Check sheet for the drawn part. Datum: minimum x, y, z corner. Units: mm. A direction names the side the tool comes from. Coordinates: 2 decimals unless noted, no trailing zeros. Loops run counter-clockwise (first coordinate to the right, second up) from the corner with the lowest first, then second, coordinate; pieces in that order, holes last.
Q1. Material ranges on probe 1 along Y at (x, z) = (10, 1.4); probe 2 along Z at (x, y) = (5, 16.5); probe 3 along Y at (x, z) = (3, 0.55), recorded low to high.
Q2. Sectioned sample at D-D (z = 1.75). Enter the section's corners in (x, y), then the cut area to 3 significant figures.
Q3. Mould release check, pull along X, two halves, no side actions. Record for the marked faces 1, 2 and 3: +X half, -X half, draft (parallel to the pull), parting line (faces both ways), or undercut.
Q4. Sectioned sample at C-C (y = 16.5). Enter the section's corners in (x, z).
Q5. Sectioned sample at A-A (x = 10). Enter the section's corners in (y, z), then the cut area to 3 significant figures.
Q6. Go/stop test with flat-tipped pins: P1, Ø2.5, axis at x = 10, y = 10, coming from the +Z side; P2, Ø1, axis at y = 14.5, z = 2, coming from the -X side. Record where each tip stops, or that it passes through.
Q7. Access from +Z, -Z, +X, -X, +Y, -Y to the whole of each face (thin tool, end or side, straight path). Record for the marked faces 4 and 5.
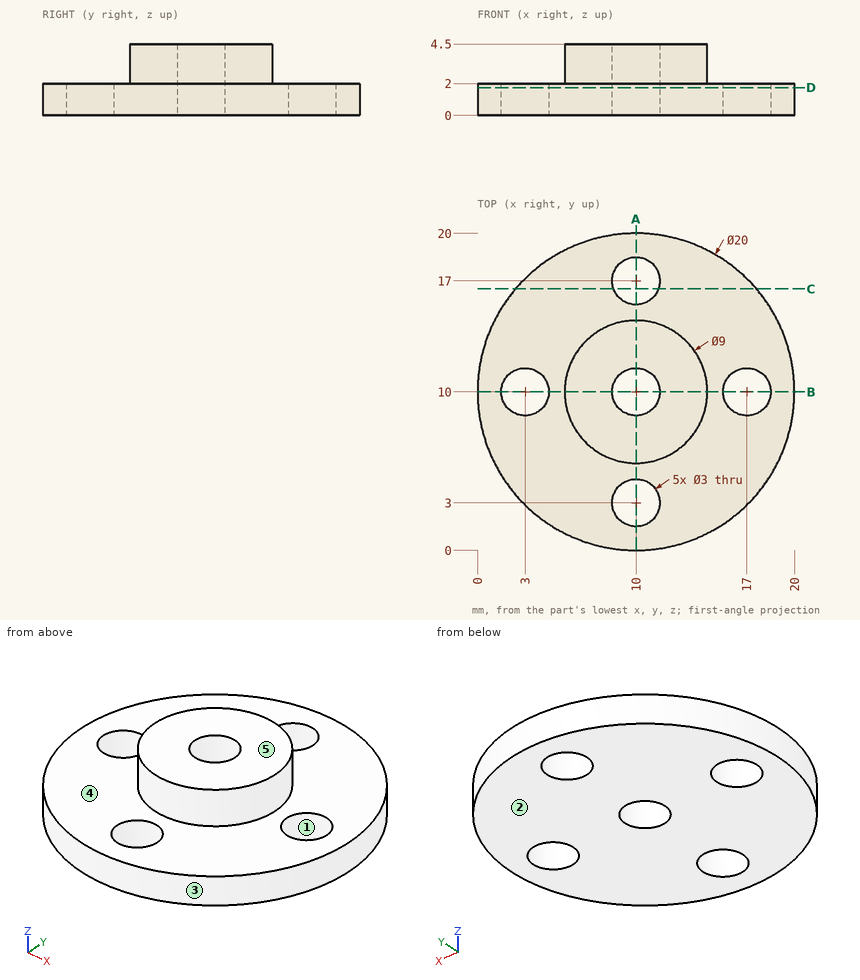
Geometry check:
1. probe 1: y = 0 to 1.5, 4.5 to 8.5, 11.5 to 15.5, 18.5 to 20
1. probe 2: z = 0 to 2
1. probe 3: y = 2.86 to 8.5, 11.5 to 17.14
2. outline: circle Ø20 at (10, 10); hole circle Ø3 at (3, 10); hole circle Ø3 at (10, 3); hole circle Ø3 at (10, 10); hole circle Ø3 at (10, 17); hole circle Ø3 at (17, 10)
2. area: 279 mm2
3. face 1: undercut
3. face 2: draft
3. face 3: parting line
4. outline: (2.4, 0) - (8.59, 0) - (8.59, 2) - (2.4, 2) - close; (11.41, 0) - (17.6, 0) - (17.6, 2) - (11.41, 2) - close
5. outline: (0, 0) - (1.5, 0) - (1.5, 2) - (0, 2) - close; (4.5, 0) - (8.5, 0) - (8.5, 4.5) - (5.5, 4.5) - (5.5, 2) - (4.5, 2) - close; (11.5, 0) - (15.5, 0) - (15.5, 2) - (14.5, 2) - (14.5, 4.5) - (11.5, 4.5) - close; (18.5, 0) - (20, 0) - (20, 2) - (18.5, 2) - close
5. area: 37.0 mm2
6. P1: passes through
6. P2: stops at x = 0.83
7. face 4: +Z
7. face 5: +Z, +X, -X, +Y, -Y
